Geometry: final body of the model. Coordinates: model frame, mm. Face numbers are marked on the shaded views. A direction names the side the tool comes from. Round coordinates to 2 decimals unless told otherwise and drop trailing zeros. Loops run counter-clockwise (first coordinate to the right, second up) from the corner with the lowest first, then second, coordinate; pieces in that order, holes last. Notation, with made-up numbers: (-35.75, 46.25) - (-25.75, 46.25) arc R16 cw to (-25.75, 55.25) - close; hole circle Ø9 at (-22, 71). An arc over 180 degrees is marked (long way). Use CSV: the item, a comma, the result in double quotes.
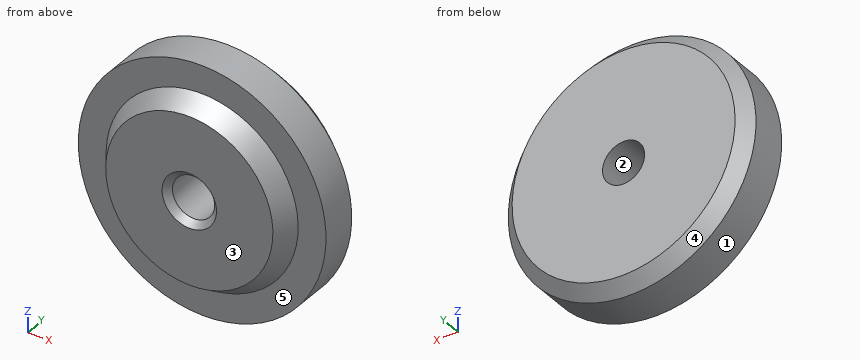
from build123d import *

# Parameters (mm, degrees)
M8_TAPPED_HOLE1_D     = 6.8
M8_TAPPED_HOLE1_DEPTH = 21.25
CHAMFER1_SIZE         = 1


with BuildPart() as part:
    # Sketch1 → Revolve1 (revolve)
    with BuildSketch(Plane.XY, mode=Mode.PRIVATE) as revolve1_sk:
        Polygon((0, 0), (0, 11), (18, 11), (20, 9), (20, 3), (15.5, 3), (13.5, 0), align=None)
    revolve(revolve1_sk.sketch.rotate(Axis((0, 0, 0), (0, 1, 0)), 90), axis=Axis((0, 0, 0), (0, 1, 0)))

    # M8 Tapped Hole1
    with Locations(Plane(origin=(0, 11, 0), x_dir=(1, 0, 0), z_dir=(0, 1, 0))):
        with Locations((0, 0)):
            Hole(M8_TAPPED_HOLE1_D / 2, depth=M8_TAPPED_HOLE1_DEPTH)

    # Chamfer1
    chamfer1_edges = [part.edges().sort_by_distance(p)[0] for p in [
        (3.4, 0, 0),
    ]]
    chamfer(chamfer1_edges, length=CHAMFER1_SIZE)


solid = part.part
Item 1: Section B-B on x = 0. Return the cut outline in (y, z), plus the area to 3 significant figures.
Final values:
outline,"(0, -13.5) - (3, -15.5) - (3, -20) - (9, -20) - (11, -18) - (11, -3.4) - (1, -3.4) - (0, -4.4) - close; (0, 4.4) - (1, 3.4) - (11, 3.4) - (11, 18) - (9, 20) - (3, 20) - (3, 15.5) - (0, 13.5) - close"
area,"327 mm²"
Item 2: Material intervals for line 1 (X direction, y = 3.5, z = 0); line 2 (X direction, y = 4, z = 2); line 3 (Y direction, x = 5, z = 17), sorted ascending.
Final values:
line 1,"x = -20 to -3.4, 3.4 to 20"
line 2,"x = -19.9 to -2.75, 2.75 to 19.9"
line 3,"y = 3 to 11"
Item 3: Section C-C on y = 4.5. Return the cut outline in (x, z), plus the area to 3 significant figures.
Final values:
outline,"circle Ø40 at (0, 0); hole circle Ø6.8 at (0, 0)"
area,"1,220 mm²"
Item 4: Reachability of the marked faces 4 and 5 from +Z, -Z, +X, -X, +Y, -Y: full face, straight path, thin tool, end or side. Return the list, or none.
Final values:
face 4,"+Y"
face 5,"-Y"
Item 5: Pin query (flat end, axial travel): P1, Ø4, axis at y = 1.5, z = 3, coming from the -X side; P2, Ø1, axis at y = 9.5, z = 12.5, coming from the +X side; P3, Ø6, axis at x = 6, y = 8.5, coming from the -Z side; P4, Ø6, axis at x = -7.5, z = 0.5, coming from the -Y side. Return the tip coordinate at first contact, or that it passes through.
Final values:
P1,"stops at x = -19.93"
P2,"stops at x = 15.72"
P3,"stops at z = -19.77"
P4,"stops at y = 0"
Item 6: Section A-A on z = 0. Return the cut outline in (x, y).
Final values:
outline,"(-20, 3) - (-15.5, 3) - (-13.5, 0) - (-4.4, 0) - (-3.4, 1) - (-3.4, 11) - (-18, 11) - (-20, 9) - close; (3.4, 1) - (4.4, 0) - (13.5, 0) - (15.5, 3) - (20, 3) - (20, 9) - (18, 11) - (3.4, 11) - close"
Item 7: Mould query, pull axis X, two halves, no side actions, for the marked faces 1, 2 and 3. Classes: released by +X, released by -X, zero draft, split by the parting line, or undercut.
Final values:
face 1,"split by the parting line"
face 2,"undercut"
face 3,"zero draft"
